Autodesk Fusion 360 part; units mm, degrees
sketch "Sketch1" plane through (0, 0, 0) normal (0, 0, 1) x (1, 0, 0)
  line L0 (8.9904, 12.5053) -> (41.0904, 12.5053)
  line L1 (41.0904, 12.5053) -> (41.0904, 60.5053)
  line L2 (41.0904, 60.5053) -> (8.9904, 60.5053)
  line L3 (8.9904, 60.5053) -> (8.9904, 12.5053)
  line L4 (41.0904, 60.5053) -> (8.9904, 60.5053)
  line L5 (8.9904, 60.5053) -> (8.9904, 12.5053)
  line L6 (8.9904, 12.5053) -> (41.0904, 12.5053)
  line L7 (41.0904, 12.5053) -> (41.0904, 60.5053)
  line L8 (8.9904, 12.5053) -> (41.0904, 12.5053)
  line L9 (41.0904, 12.5053) -> (41.0904, 60.5053)
  line L10 (41.0904, 60.5053) -> (8.9904, 60.5053)
  line L11 (8.9904, 60.5053) -> (8.9904, 12.5053)
  line L12 (8.9904, 12.5053) -> (13.0904, 12.5053)
  line L13 (13.0904, 12.5053) -> (13.0904, 16.5053)
  line L14 (13.0904, 16.5053) -> (8.9904, 16.5053)
  line L15 (8.9904, 16.5053) -> (8.9904, 12.5053)
  line L16 (41.0904, 12.5053) -> (36.9904, 12.5053)
  line L17 (36.9904, 12.5053) -> (36.9904, 16.5053)
  line L18 (36.9904, 16.5053) -> (41.0904, 16.5053)
  line L19 (41.0904, 16.5053) -> (41.0904, 12.5053)
  line L20 (8.9904, 12.5053) -> (25.0404, 12.5053)
  line L21 (25.0404, 12.5053) -> (25.0404, 36.5053)
  line L22 (25.0404, 36.5053) -> (8.9904, 36.5053)
  line L23 (8.9904, 36.5053) -> (8.9904, 12.5053)
  circle A0 centre (25.0404, 36.5053) radius 2.25
  line L24 (25.0404, 12.5053) -> (28.5404, 12.5053)
  line L25 (28.5404, 12.5053) -> (28.5404, 17.8053)
  line L26 (28.5404, 17.8053) -> (25.0404, 17.8053)
  line L27 (25.0404, 17.8053) -> (25.0404, 12.5053)
  line L28 (25.0404, 12.5053) -> (21.5404, 12.5053)
  line L29 (21.5404, 12.5053) -> (21.5404, 17.8053)
  line L30 (21.5404, 17.8053) -> (25.0404, 17.8053)
  line L31 (25.0404, 17.8053) -> (25.0404, 12.5053)
  circle A1 centre (12.9235, 34.5524) radius 1.625
  circle A2 centre (12.9235, 46.5524) radius 1.625
  circle A3 centre (12.9235, 56.5524) radius 1.625
  circle A4 centre (36.8235, 56.5524) radius 1.625
  circle A5 centre (36.8235, 46.5524) radius 1.625
  circle A6 centre (36.8235, 34.5524) radius 1.625
  circle A7 centre (36.9904, 16.5053) radius 1.625
  circle A8 centre (13.0904, 16.5053) radius 1.625
  circle A9 centre (25.0404, 36.5053) radius 3.75
  point P0 (12.9235, 16.5524)
  dimension "d1" = 32.1
  dimension "d2" = 48
  dimension "d5" = 4.1
  dimension "d6" = 4
  dimension "d8" = 4.1
  dimension "d9" = 4
  dimension "d17" = 16.05
  dimension "d18" = 24
  dimension "d20" = 4.5
  dimension "d21" = 3.5
  dimension "d22" = 5.3
  dimension "d23" = 3.5
  dimension "d24" = 5.3
  dimension "d31" = 3.25
  dimension "d32" = 3.25
  dimension "d33" = 3.25
  dimension "d34" = 3.25
  dimension "d35" = 3.25
  dimension "d36" = 3.25
  dimension "d37" = 3.25
  dimension "d38" = 3.25
  dimension "d45" = 7.5
extrude "Extrude8" add sketch "Sketch1" along normal blind 7 contours L0 L3 L5 L6 L8 L11 L12 L13 L14 L15 L20 L23 A8 | L0 L3 L5 L6 L8 L11 L13 L14 L20 L21 L22 L23 L29 L30 A8 A9 | L0 L1 L2 L3 L4 L5 L6 L7 L8 L9 L10 L11 L17 L18 L21 L22 L25 L26 A7 A9 | L0 L1 L6 L7 L8 L9 L16 L17 L18 L19 A7
extrude "Extrude9" add sketch "Sketch1" along normal blind 5.5 contours L0 L6 L8 L20 L21 L27 L28 L29 L30 L31 | L0 L6 L8 L21 L24 L25 L26 L27 L31
extrude "Extrude10" add sketch "Sketch1" along normal blind 2.5 contours L21 L22 A0 A9 | L21 L22 A0 A9
Design review of the part built by this model. Coordinates are the model's own, in mm. A direction names the side the tool comes from. Round coordinates to 2 decimals unless told otherwise and drop trailing zeros. Write each loop counter-clockwise with the first axis right and the second up, starting at its lowest first coordinate (ties: lowest second). Pieces come first, ordered by that corner, then holes. Notation, with made-up numbers: (-21.75, -23) - (34.25, -23) arc R14 cw to (34.25, -18) - close; hole circle Ø10 at (-12.5, 62.25). An arc over 180 degrees is marked (long way). Return JSON: item names as keys, results as strings. Group by question number.
Item 1: We need section A-A on y = 33.5. Write out the cut boundary in (x, z).
Item 2: Insertion check: P1, Ø6, axis at x = 17.5, y = 55, coming from the -Z side; P2, Ø3, axis at x = 12.92, y = 46.55, coming from the -Z side; P3, Ø3, axis at x = 24, y = 36, coming from the +Z side; P4, Ø1.2, axis at x = 26.5, z = 6.5, coming from the -Y side. Each pin has a flat end and moves straight along its axis. Give the tip position at first contact, or say it passes through.
Item 3: We need section D-D on x = 23.5. Write out the cut boundary in (y, z).
Item 4: Machinability: for faces 1 (the face through (25, 15, 5.5)), 2 (the face through (36.47, 58.14, 3.45)), 3 (the face through (27, 35, 2.5)), which of the approach directions +Z, -Z, +X, -X, +Y, -Y give a long, thin tool a straight path to every point of the face, cutting with its end or side? Answer none if there is none.
Item 5: For probe 1 along Y at (x, z) = (12, 6.25); probe 2 along Y at (x, z) = (27, 1); probe 3 along Y at (x, z) = (24.5, 4.5), list the stretches that pass through material, from the lowest coordinate up. Write a range as [from, to].
Item 6: We need section B-B on z = 4.75. Give the number of separate pieces and of enclosed holes in the cut face, and give its area (3 significant figures).
Item 7: We need section C-C on x = 36.5. Write out the cut boundary in (y, z).
Item 8: The part is to be moulded in two halves that separate along Y. For faces 4 (the face through (38.54, 16.02, 3.45)), 5 (the face through (25, 12.505, 3)), 6 (the face through (28, 37, 0)), say which applies: pulls with the +Y half, pulls with the -Y half, needs draft (parallel to the pull), parting line crosses it, or undercut.
Model answer:
{
 "1": {"outline": "(8.99, 0) - (11.69, 0) - (11.69, 7) - (8.99, 7) - close; (14.16, 0) - (35.59, 0) - (35.59, 7) - (27.28, 7) - (27.28, 2.5) - (22.8, 2.5) - (22.8, 7) - (14.16, 7) - close; (38.06, 0) - (41.09, 0) - (41.09, 7) - (38.06, 7) - close"},
 "2": {"P1": "stops at z = 0", "P2": "passes through", "P3": "stops at z = 2.5", "P4": "stops at y = 17.81"},
 "3": {"outline": "(12.51, 0) - (34.87, 0) - (34.87, 2.5) - (33.09, 2.5) - (33.09, 7) - (17.81, 7) - (17.81, 5.5) - (12.51, 5.5) - close; (38.15, 0) - (60.51, 0) - (60.51, 7) - (39.92, 7) - (39.92, 2.5) - (38.15, 2.5) - close"},
 "4": {"face 1": "+Z, -Y", "face 2": "+Z, -Z", "face 3": "+Z"},
 "5": {"probe 1": "y = [12.51, 15.3], [17.71, 33.22], [35.89, 45.22], [47.89, 55.22], [57.89, 60.51]", "probe 2": "y = [12.51, 35.4], [37.61, 60.51]", "probe 3": "y = [12.51, 32.79], [40.22, 60.51]"},
 "6": {"separate pieces": "1", "enclosed holes": "9", "area": "1,430 mm²"},
 "7": {"outline": "(12.51, 0) - (14.96, 0) - (14.96, 7) - (12.51, 7) - close; (18.05, 0) - (32.96, 0) - (32.96, 7) - (18.05, 7) - close; (36.14, 0) - (44.96, 0) - (44.96, 7) - (36.14, 7) - close; (48.14, 0) - (54.96, 0) - (54.96, 7) - (48.14, 7) - close; (58.14, 0) - (60.51, 0) - (60.51, 7) - (58.14, 7) - close"},
 "8": {"face 4": "undercut", "face 5": "pulls with the -Y half", "face 6": "needs draft"}
}
